CAD build for the part. Positions are in the model's coordinates, mm. Face numbers are marked on the shaded views. A direction names the side the tool comes from. Coordinates: 2 decimals unless noted, no trailing zeros. Order: outer loops, then holes, each group sorted by start corner. A loop starts at its lowest first (then second) coordinate and runs counter-clockwise, first axis right, second up. Notation, with made-up numbers: M 74,16 L 105,16 A20 cw 105,33 Z; hole C 86,48 d8. An arc over 180 degrees is marked long. Write item = value, one per line.
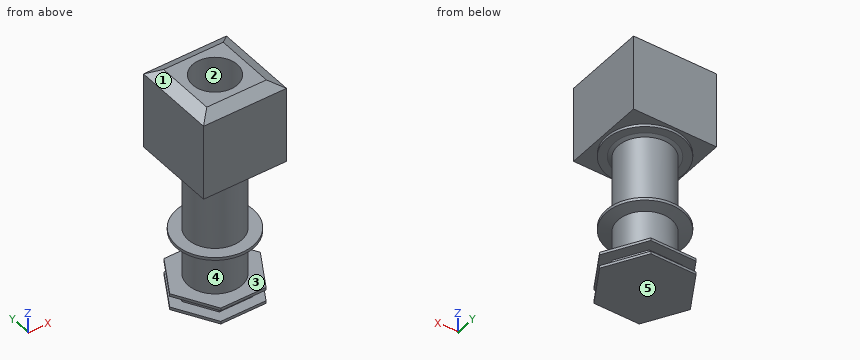
from build123d import *
from OCP.BRepFilletAPI import BRepFilletAPI_MakeChamfer

# Parameters (mm, degrees)
BOSS_EXTRUDE1_DEPTH = 12
BOSS_EXTRUDE2_DEPTH = 50
BOSS_EXTRUDE3_DEPTH = 12
SKETCH4_R           = 120
BOSS_EXTRUDE4_DEPTH = 200
SKETCH5_R           = 172.646944325
BOSS_EXTRUDE5_DEPTH = 12
CHAMFER1_SIZE       = 56.712818196
CHAMFER1_SIZE_2     = 10
SKETCH6_R           = 120
BOSS_EXTRUDE6_DEPTH = 330
SKETCH8_R           = 172.646944325
BOSS_EXTRUDE7_DEPTH = 12
CHAMFER2_SIZE       = 6
CHAMFER2_SIZE2      = 16.484864517
SKETCH9_W           = 370
SKETCH9_H           = 370
BOSS_EXTRUDE8_DEPTH = 370
SKETCH10_R          = 100
CUT_EXTRUDE1_DEPTH  = 900
CHAMFER3_SIZE       = 30
CHAMFER3_SIZE2      = 51.961524227


with BuildPart() as part:
    # Sketch1 → Boss-Extrude1 (new body)
    with BuildSketch(Plane.XY):
        Polygon((202.072594216, 0), (101.036297108, 175), (-101.036297108, 175), (-202.072594216, 0), (-101.036297108, -175), (101.036297108, -175), align=None)
    extrude(amount=BOSS_EXTRUDE1_DEPTH)

    # Sketch2 → Boss-Extrude2 (add)
    with BuildSketch(Plane.XY.offset(12)):
        Polygon((147.887498821, 0), (73.943749411, 128.074330881), (-73.943749411, 128.074330881), (-147.887498821, 0), (-73.943749411, -128.074330881), (73.943749411, -128.074330881), align=None)
    extrude(amount=BOSS_EXTRUDE2_DEPTH)

    # Sketch3 → Boss-Extrude3 (add)
    with BuildSketch(Plane.XY.offset(62)):
        Polygon((202.072594216, 0), (101.036297108, 175), (-101.036297108, 175), (-202.072594216, 0), (-101.036297108, -175), (101.036297108, -175), align=None)
    extrude(amount=BOSS_EXTRUDE3_DEPTH)

    # Sketch4 → Boss-Extrude4 (add)
    with BuildSketch(Plane.XY.offset(74)):
        Circle(SKETCH4_R)
    extrude(amount=BOSS_EXTRUDE4_DEPTH)

    # Sketch5 → Boss-Extrude5 (add)
    with BuildSketch(Plane.XY.offset(274)):
        Circle(SKETCH5_R)
    extrude(amount=BOSS_EXTRUDE5_DEPTH)

    # Chamfer1
    # the kernel refuses this chamfer: 56.712818196, 10 mm, written as the material it adds along each edge
    with BuildSketch(Plane(origin=(0, 0, 274), x_dir=(1, 0, 0), z_dir=(0, -1, 0))) as chamfer1_piece_1_section:
        Polygon((120 + CHAMFER1_SIZE, 0), (120, -CHAMFER1_SIZE_2), (120, 0), align=None)
    chamfer1_piece_1 = revolve(axis=Axis((0, 0, 274), (0, 0, 1)), mode=Mode.PRIVATE)
    chamfer1_piece_1 = chamfer1_piece_1 & Plane(origin=(0, 0, 269.114385433), x_dir=(1, 0, 0), z_dir=(0, 0, -1)) * Cylinder(172.646944325, 707, mode=Mode.PRIVATE)
    add(chamfer1_piece_1)

    # Sketch6 → Boss-Extrude6 (add)
    with BuildSketch(Plane.XY.offset(286)):
        Circle(SKETCH6_R)
    extrude(amount=BOSS_EXTRUDE6_DEPTH)

    # Sketch8 → Boss-Extrude7 (add)
    with BuildSketch(Plane.XY.offset(616)):
        Circle(SKETCH8_R)
    extrude(amount=BOSS_EXTRUDE7_DEPTH)

    # Chamfer2
    chamfer2_edges = [part.edges().sort_by_distance(p)[0] for p in [
        (-120, 0, 616),
    ]]
    chamfer2_side = [part.faces().sort_by_distance(p)[0] for p in [
        (-120, 0, 451),
    ]]
    chamfer(chamfer2_edges, length=CHAMFER2_SIZE, length2=CHAMFER2_SIZE2, reference=chamfer2_side[0])

    # Sketch9 → Boss-Extrude8 (add)
    with BuildSketch(Plane.XY.offset(628)):
        Rectangle(SKETCH9_W, SKETCH9_H)
    extrude(amount=BOSS_EXTRUDE8_DEPTH)

    # Sketch10 → Cut-Extrude1 (cut)
    with BuildSketch(Plane.XY.offset(998)):
        Circle(SKETCH10_R)
    extrude(amount=-CUT_EXTRUDE1_DEPTH, mode=Mode.SUBTRACT)

    # Chamfer3: one chamfer whose edges measure the first distance from different faces: ONE call of the kernel's chamfer builder (chamfer() names one face for all edges)
    chamfer3_edges_1 = [part.edges().sort_by_distance(p)[0] for p in [
        (185, 0, 998),
    ]]
    chamfer3_side_1 = [part.faces().sort_by_distance(p)[0] for p in [
        (185, 0, 813),
    ]]
    chamfer3_edges_2 = [part.edges().sort_by_distance(p)[0] for p in [
        (0, 185, 998),
    ]]
    chamfer3_side_2 = [part.faces().sort_by_distance(p)[0] for p in [
        (0, 185, 813),
    ]]
    chamfer3_edges_3 = [part.edges().sort_by_distance(p)[0] for p in [
        (-185, 0, 998),
    ]]
    chamfer3_side_3 = [part.faces().sort_by_distance(p)[0] for p in [
        (-185, 0, 813),
    ]]
    chamfer3_edges_4 = [part.edges().sort_by_distance(p)[0] for p in [
        (0, -185, 998),
    ]]
    chamfer3_side_4 = [part.faces().sort_by_distance(p)[0] for p in [
        (0, -185, 813),
    ]]
    chamfer3 = BRepFilletAPI_MakeChamfer(part.part.solid().wrapped)
    for e in chamfer3_edges_1:
        chamfer3.Add(CHAMFER3_SIZE, CHAMFER3_SIZE2, e.wrapped, chamfer3_side_1[0].wrapped)  # the first distance lies on this face
    for e in chamfer3_edges_2:
        chamfer3.Add(CHAMFER3_SIZE, CHAMFER3_SIZE2, e.wrapped, chamfer3_side_2[0].wrapped)  # the first distance lies on this face
    for e in chamfer3_edges_3:
        chamfer3.Add(CHAMFER3_SIZE, CHAMFER3_SIZE2, e.wrapped, chamfer3_side_3[0].wrapped)  # the first distance lies on this face
    for e in chamfer3_edges_4:
        chamfer3.Add(CHAMFER3_SIZE, CHAMFER3_SIZE2, e.wrapped, chamfer3_side_4[0].wrapped)  # the first distance lies on this face
    add(Compound.cast(chamfer3.Shape()), mode=Mode.REPLACE)


solid = part.part
(1) Pin check, flat tips, straight feed: pin 1 Ø13 at (x, z) = (-41, 66) entering from +Y; pin 2 Ø12 at (y, z) = (91, 247) entering from +X; pin 3 Ø1 at (x, z) = (98.5, 181) entering from +Y. Stop position of each tip, or through.
Evaluation:
pin_1 = 175
pin_2 = 84.71
pin_3 = 69.25
(2) Slice it at A-A, the plane z = 701. Write the cut outline in (x, y).
Evaluation:
outline = M -185,-185 L 185,-185 L 185,185 L -185,185 Z; hole C 0,0 d200
(3) Slice it at B-B, the plane z = 513. Write the cut outline in (x, y).
Evaluation:
outline = C 0,0 d240; hole C 0,0 d200
(4) Tool access for the marked faces 4 and 5: list every direction of +Z, -Z, +X, -X, +Y, -Y with a clear straight run to the whole face (end or side of a thin tool).
Evaluation:
face_4 = none
face_5 = -Z, +X, -X, +Y, -Y
(5) Pull direction X, two halves, no side cores. Call the marked faces 1, 2 and 3: +X half, -X half, draft (parallel to the pull), parting line (faces both ways), or undercut.
Evaluation:
face_1 = -X half
face_2 = undercut
face_3 = draft
(6) Wall check: line 1 (Y direction, x = 0, z = 446); line 2 (Y direction, x = 0, z = 794.5); line 3 (Z direction, x = -108.5, y = -54.5). Give the ranges that are in metal, low to high. Write a range as from..to.
Evaluation:
line_1 = -120..-100, 100..120
line_2 = -185..-100, 100..185
line_3 = 0..74, 264.25..286, 610.52..998
